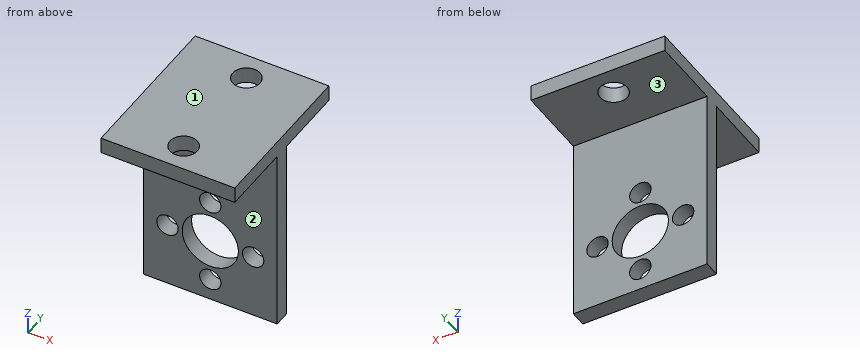
Autodesk Inventor part; units mm, degrees
ref_plane "YZ Plane" through (0, 0, 0) normal (1, 0, 0) x (0, 1, 0)
ref_plane "XZ Plane" through (0, 0, 0) normal (0, 1, 0) x (-1, 0, 0)
ref_plane "XY Plane" through (0, 0, 0) normal (0, 0, 1) x (1, 0, 0)
sketch "Sketch1" plane through (0, 0, 0) normal (0, 0, 1) x (1, 0, 0)
  line L0 (12.5, 15) -> (-12.5, 15)
  line L1 (-12.5, 15) -> (-12.5, -15)
  line L2 (-12.5, -15) -> (12.5, -15)
  line L3 (12.5, -15) -> (12.5, 15)
  line L4 (12.5, 15) -> (-12.5, -15) construction
  line L5 (-12.5, 15) -> (12.5, -15) construction
  point P0 (0, 0)
  dimension "d0" = 25
  dimension "d1" = 30
extrude "Extrusion1" add sketch "Sketch1" against normal blind 3
sketch "Sketch2" plane through (0, 0, -3) normal (0, 0, -1) x (-1, 0, 0)
  line L0 (12.5, -15) -> (12.5, 15)
  line L1 (-12.5, 1.5) -> (12.5, 1.5)
  line L2 (12.5, 1.5) -> (12.5, -1.5)
  line L3 (12.5, -1.5) -> (-12.5, -1.5)
  line L4 (-12.5, -1.5) -> (-12.5, 1.5)
  line L5 (-12.5, 1.5) -> (12.5, -1.5) construction
  line L6 (12.5, 1.5) -> (-12.5, -1.5) construction
  point P0 (0, 0)
  dimension "d4" = 3
extrude "Extrusion2" add sketch "Sketch2" along normal blind 35
sketch "Sketch3" plane through (0, 0, 0) normal (0, 0, 1) x (1, 0, 0)
  line L0 (0, 10) -> (0, -10)
  circle A0 centre (0, 10) radius 2.55
  circle A1 centre (0, -10) radius 2.55
  point P0 (0, 0)
  dimension "d7" = 20
  dimension "d8" = 5.1
  dimension "d9" = 5.1
extrude "Extrusion3" cut sketch "Sketch3" against normal through all
sketch "Sketch4" plane through (-12.5, 1.5, -3) normal (0, 1, 0) x (1, 0, 0)
  line L0 (9.95, 0) -> (15.05, 0)
  line L1 (12.5, 0) -> (12.5, 22.896)
  circle A0 centre (12.5, 22.896) radius 5.25
  circle A1 centre (12.5, 22.896) radius 8
  circle A2 centre (12.5, 14.896) radius 2
  circle A3 centre (20.5, 22.896) radius 2
  circle A4 centre (12.5, 30.896) radius 2
  circle A5 centre (4.5, 22.896) radius 2
  point P0 (12.5, -3)
  dimension "d14" = 16
  dimension "d12" = 22.896
  dimension "d13" = 10.5
  dimension "d15" = 4
  dimension "d18" = 360
extrude "Extrusion4" cut sketch "Sketch4" against normal through all contours A2 A1 L1 | L1 A1 A2 | A1 A2 L1 | L1 A2 A1 | A0 | A5 A1 | A1 A5 | A3 A1 | A1 A3 | A4 A1 | A1 A4
properties part number "LeadCarriageConnector"
Model file for the job. Use its own axes, mm. Face numbers are marked on the shaded views. A direction names the side the tool comes from. Round coordinates to 2 decimals unless told otherwise and drop trailing zeros. Order: outer loops, then holes, each group sorted by start corner. A loop starts at its lowest first (then second) coordinate and runs counter-clockwise, first axis right, second up. Notation, with made-up numbers: (-7.5, -34.5) -> (33.5, -34.5) arc R21 ccw to (33.5, -24.5) -> close; hole circle Ø11 at (44.5, 57). An arc over 180 degrees is marked (long way). Use one line per item in the form item = value.
Item 1: Cut at B-B, the plane x = 8. Write the cut outline in (y, z), and give its area (3 significant figures).
Returned:
outline = (-15, -3) -> (-1.5, -3) -> (-1.5, -23.9) -> (1.5, -23.9) -> (1.5, -3) -> (15, -3) -> (15, 0) -> (-15, 0) -> close; (-1.5, -38) -> (1.5, -38) -> (1.5, -27.9) -> (-1.5, -27.9) -> close
area = 183 mm^2
Item 2: Cut at D-D, the plane z = -29.5. Write the cut outline in (x, y), and give its area (3 significant figures).
Returned:
outline = (-12.5, -1.5) -> (-3.82, -1.5) -> (-3.82, 1.5) -> (-12.5, 1.5) -> close; (3.82, -1.5) -> (12.5, -1.5) -> (12.5, 1.5) -> (3.82, 1.5) -> close
area = 52.1 mm^2
Item 3: Flat gauge pins, fed straight in: pin 1 Ø6 at (x, z) = (0, -10.5) entering from -Y; pin 2 Ø3.5 at (x, z) = (8, -25.896) entering from -Y; pin 3 Ø4.5 at (x, z) = (0, -33.896) entering from +Y; pin 4 Ø15 at (x, y) = (-5, -11.5) entering from -Z. Where does each tip first touch, or does it go through?
Returned:
pin_1 = -1.5
pin_2 = through
pin_3 = 1.5
pin_4 = -3
Item 4: Tool access for the marked faces 1, 2 and 3: list every direction of +Z, -Z, +X, -X, +Y, -Y with a clear straight run to the whole face (end or side of a thin tool).
Returned:
face_1 = +Z, +X, -X, +Y, -Y
face_2 = -Z, +X, -X, -Y
face_3 = -Z, +X, -X, +Y
Item 5: Drill centre lines: line 1 (Z direction, x = 0, y = 0); line 2 (X direction, y = -10, z = -1.65); line 3 (Y direction, x = 6, z = -22). Where is each one in solid material? Low to high.
Returned:
line_1 = -38 to -35.9, -31.9 to -31.15, -20.65 to -19.9, -15.9 to 0
line_2 = -12.5 to -2.55, 2.55 to 12.5
line_3 = -1.5 to 1.5
Item 6: Cut at C-C, the plane x = 0. Write the cut outline in (y, z), and give its area (3 significant figures).
Returned:
outline = (-15, -3) -> (-12.55, -3) -> (-12.55, 0) -> (-15, 0) -> close; (-7.45, -3) -> (-1.5, -3) -> (-1.5, -15.9) -> (1.5, -15.9) -> (1.5, -3) -> (7.45, -3) -> (7.45, 0) -> (-7.45, 0) -> close; (-1.5, -38) -> (1.5, -38) -> (1.5, -35.9) -> (-1.5, -35.9) -> close; (-1.5, -31.9) -> (1.5, -31.9) -> (1.5, -31.15) -> (-1.5, -31.15) -> close; (-1.5, -20.65) -> (1.5, -20.65) -> (1.5, -19.9) -> (-1.5, -19.9) -> close; (12.55, -3) -> (15, -3) -> (15, 0) -> (12.55, 0) -> close
area = 109 mm^2
Item 7: Cut at A-A, the plane y = 10. Write the cut outline in (x, z), and give its area (3 significant figures).
Returned:
outline = (-12.5, -3) -> (-2.55, -3) -> (-2.55, 0) -> (-12.5, 0) -> close; (2.55, -3) -> (12.5, -3) -> (12.5, 0) -> (2.55, 0) -> close
area = 59.7 mm^2
